Autodesk Inventor part; units mm, degrees
ref_plane "YZ Plane" through (0, 0, 0) normal (1, 0, 0) x (0, 1, 0)
ref_plane "XZ Plane" through (0, 0, 0) normal (0, 1, 0) x (-1, 0, 0)
ref_plane "XY Plane" through (0, 0, 0) normal (0, 0, 1) x (1, 0, 0)
sketch "Boceto1" plane through (0, 0, 0) normal (0, 1, 0) x (-1, 0, 0)
  line L0 (10, 0) -> (10, -26.35)
  line L1 (0, -26.35) -> (0, 0)
  line L2 (0, 0) -> (0, 3)
  line L3 (0, 3) -> (10, 3)
  line L4 (10, 3) -> (10, 0)
  line L5 (10, -26.35) -> (10, -29.35)
  line L6 (10, -29.35) -> (0, -29.35)
  line L7 (0, -29.35) -> (0, -26.35)
extrude "Extrusión1" add sketch "Boceto1" along normal blind 3
sketch "Boceto3" plane through (0, 0, 0) normal (0, -1, 0) x (1, 0, 0)
  line L0 (0, 3) -> (0, 6)
  line L1 (0, 6) -> (-7, 6)
  line L2 (-7, 6) -> (-7, 3)
  line L3 (-7, 3) -> (0, 3)
  line L4 (0, -29.35) -> (0, -32.35)
  line L5 (0, -32.35) -> (-7, -32.35)
  line L6 (-7, -32.35) -> (-7, -29.35)
  line L7 (0, -29.35) -> (-7, -29.35)
  point P0 (0, 0)
extrude "Extrusión3" add sketch "Boceto3" against normal blind 3
properties part number "muñeca2"
The model under review builds one solid part; all positions refer to its coordinate system, in mm. A direction names the side the tool comes from. Coordinates: 2 decimals unless noted, no trailing zeros. Write each loop counter-clockwise with the first axis right and the second up, starting at its lowest first coordinate (ties: lowest second). Pieces come first, ordered by that corner, then holes. Notation, with made-up numbers: (80.25, -39) - (136.25, -39) arc R18 cw to (136.25, -18) - close; hole circle Ø6 at (37.25, 68.5). An arc over 180 degrees is marked (long way). Answer as CSV lines item,"result".
(1) For line 1 along Z through (x, y) = (-7.75, 1.15), list the stretches that pass through material, from the lowest coordinate up. Write a range as [from, to].
Data:
line 1,"z = [-29.35, 3]"
(2) Clearance check with a flat-ended pin moving along its axis: pin 1 Ø1.5 at (x, y) = (-9, 1.5) entering from +Z. State where the tip first meets the part, or that it passes through.
Data:
pin 1,"stops at z = 3"
(3) We need section B-B (x = -9). Give the boundary of the cut face in (y, z).
Data:
outline,"(0, -29.35) - (3, -29.35) - (3, 3) - (0, 3) - close"
(4) Tool access review of faces 1 (the flat face through (-10, 1, -13)), 2 (the flat face through (-7, 1, -31)), 3 (the flat face through (-7, 1, 5)): name each direction out of +Z, -Z, +X, -X, +Y, -Y from which nothing blocks a thin tool from reaching the whole face with its end or side.
Data:
face 1,"+Z, -Z, -X, +Y, -Y"
face 2,"-Z, -X, +Y, -Y"
face 3,"+Z, -X, +Y, -Y"
(5) We need section A-A (y = 0.6). Give the boundary of the cut face in (x, z), plus the area to 4 significant figures.
Data:
outline,"(-10, -29.35) - (-7, -29.35) - (-7, -32.35) - (0, -32.35) - (0, 6) - (-7, 6) - (-7, 3) - (-10, 3) - close"
area,"365.5 mm2"
